```python
from build123d import *

# Parameters (mm, degrees)
SKETCH1_R                                    = 27
BOSS_EXTRUDE1_DEPTH                          = 4
CBORE_FOR_M3_HEX_SOCKET_THIN_HEAD_CA_2_COUNT = 2
CBORE_FOR_M3_HEX_SOCKET_THIN_HEAD_CA_2_PITCH = 31.112698372
CBORE_FOR_M3_HEX_SOCKET_THIN_HEAD_CA_3_COUNT = 2
CBORE_FOR_M3_HEX_SOCKET_THIN_HEAD_CA_3_PITCH = 44
CBORE_FOR_M3_HEX_SOCKET_THIN_HEAD_CA_4_COUNT = 2
CBORE_FOR_M3_HEX_SOCKET_THIN_HEAD_CA_4_PITCH = 31.112698372
BOSS_EXTRUDE2_START                          = -4
BOSS_EXTRUDE2_DEPTH                          = 4
SKETCH5_R                                    = 15
CUT_EXTRUDE1_DEPTH                           = 41.558599581


with BuildPart() as part:
    # Sketch1 → Boss-Extrude1 (new body)
    with BuildSketch(Plane.XY):
        Circle(SKETCH1_R)
    extrude(amount=BOSS_EXTRUDE1_DEPTH)

    # Sketch3 → CBORE for M3 Hex Socket Thin Head Cap Screw1 (revolve, cut)
    with BuildSketch(Plane(origin=(-22, 0, 4), x_dir=(0, -1, 0), z_dir=(1, 0, 0))):
        Polygon((0, 0), (0, 4), (1.7, 4), (1.7, 2.4), (3.25, 2.4), (3.25, 0.025), (3.275, 0), align=None)
    cbore_for_m3_hex_socket_thin_head_cap_sc = revolve(axis=Axis((-22, 0, 10.35), (0, 0, -1)), mode=Mode.SUBTRACT)

    # CBORE for M3 Hex Socket Thin Head Ca 2: CBORE for M3 Hex Socket Thin Head Cap Screw1 ×2
    with Locations(*[Vector(0.7071067811865277, 0.7071067811865674, 0) * (i * CBORE_FOR_M3_HEX_SOCKET_THIN_HEAD_CA_2_PITCH) for i in range(1, CBORE_FOR_M3_HEX_SOCKET_THIN_HEAD_CA_2_COUNT)]):
        add(cbore_for_m3_hex_socket_thin_head_cap_sc, mode=Mode.SUBTRACT)

    # CBORE for M3 Hex Socket Thin Head Ca 3: CBORE for M3 Hex Socket Thin Head Cap Screw1 ×2
    with Locations(*[(i * CBORE_FOR_M3_HEX_SOCKET_THIN_HEAD_CA_3_PITCH, 0, 0) for i in range(1, CBORE_FOR_M3_HEX_SOCKET_THIN_HEAD_CA_3_COUNT)]):
        add(cbore_for_m3_hex_socket_thin_head_cap_sc, mode=Mode.SUBTRACT)

    # CBORE for M3 Hex Socket Thin Head Ca 4: CBORE for M3 Hex Socket Thin Head Cap Screw1 ×2
    with Locations(*[Vector(0.7071067811865676, -0.7071067811865276, 0) * (i * CBORE_FOR_M3_HEX_SOCKET_THIN_HEAD_CA_4_PITCH) for i in range(1, CBORE_FOR_M3_HEX_SOCKET_THIN_HEAD_CA_4_COUNT)]):
        add(cbore_for_m3_hex_socket_thin_head_cap_sc, mode=Mode.SUBTRACT)

    # Sketch4 → Boss-Extrude2 (add)
    with BuildSketch(Plane.XY.offset(4).offset(BOSS_EXTRUDE2_START)):
        with BuildLine():
            Line((-27, 0), (-27, -30))
            Line((-27, -30), (27, -30))
            Line((27, -30), (27, 0))
            ThreePointArc((27, 0), (0, -27), (-27, 0))
        make_face()
    extrude(amount=BOSS_EXTRUDE2_DEPTH)

    # Sketch5 → Cut-Extrude1 (cut, through all)
    with BuildSketch(Plane(origin=(0, 0, 0), x_dir=(-1, 0, 0), z_dir=(0, 0, -1))):
        Circle(SKETCH5_R)
    extrude(amount=-CUT_EXTRUDE1_DEPTH, mode=Mode.SUBTRACT)


solid = part.part
```
Geometry check sheet. Reference: the model listing, model coordinates, mm. A direction names the side the tool comes from. Coordinates: 2 decimals unless noted, no trailing zeros. Order: outer loops, then holes, each group sorted by start corner. A loop starts at its lowest first (then second) coordinate and runs counter-clockwise, first axis right, second up.
Q1. Thickness scan on probe 1 along Y at (x, z) = (0, 3.3); probe 2 along Y at (x, z) = (0, 0.8); probe 3 along X at (y, z) = (0.5, 1.55). Record the ranges inside material, lowest first.
Reply:
probe 1: y = -30 to -25.25, -18.75 to -15, 15 to 18.75, 25.25 to 27
probe 2: y = -30 to -23.7, -20.3 to -15, 15 to 20.3, 23.7 to 27
probe 3: x = -27 to -23.62, -20.38 to -14.99, 14.99 to 20.38, 23.62 to 27
Q2. Depth check by flat-ended pin: pin 1 Ø3 at (x, y) = (23, 0.5) entering from +Z; pin 2 Ø7.5 at (x, y) = (-22, 0) entering from +Z. Enter the tip coordinate at first touch or a pass-through.
Reply:
pin 1: stops at z = 1.6
pin 2: stops at z = 4
Q3. Tool access check on faces 4 (the face through (-6, -14, 4)), 5 (the face through (-0.98, 18.9, 2.8)). Record the directions out of +Z, -Z, +X, -X, +Y, -Y that give a thin tool (end or side, any length) a straight path to the whole face; none if there is none.
Reply:
face 4: +Z, +X, -X, +Y, -Y
face 5: +Z
Q4. Sectioned sample at C-C on x = 10.5. Record the cut outline in (y, z), and give its area (3 significant figures).
Reply:
outline: (-30, 0) - (-10.71, 0) - (-10.71, 4) - (-30, 4) - close; (10.71, 0) - (24.87, 0) - (24.87, 4) - (10.71, 4) - close
area: 134 mm2
Q5. Sectioned sample at A-A on x = 0. Record the cut outline in (y, z) (3 decimals).
Reply:
outline: (-30, 0) - (-23.7, 0) - (-23.7, 1.6) - (-25.25, 1.6) - (-25.25, 3.975) - (-25.275, 4) - (-30, 4) - close; (-20.3, 0) - (-15, 0) - (-15, 4) - (-18.725, 4) - (-18.75, 3.975) - (-18.75, 1.6) - (-20.3, 1.6) - close; (15, 0) - (20.3, 0) - (20.3, 1.6) - (18.75, 1.6) - (18.75, 3.975) - (18.725, 4) - (15, 4) - close; (23.7, 0) - (27, 0) - (27, 4) - (25.275, 4) - (25.25, 3.975) - (25.25, 1.6) - (23.7, 1.6) - close
Q6. Sectioned sample at D-D on y = 7. Record the cut outline in (x, z), and give its area (3 significant figures).
Reply:
outline: (-26.08, 0) - (-13.27, 0) - (-13.27, 4) - (-26.08, 4) - close; (13.27, 0) - (26.08, 0) - (26.08, 4) - (13.27, 4) - close
area: 102 mm2
Q7. Draft check along X on faces 1 (the face through (-0.143, -18.753, 2.804)), 2 (the face through (-6, -14, 0)), 3 (the face through (27, -15, 2)). Enter one of: released by +X, released by -X, zero draft, split by the parting line, or undercut.
Reply:
face 1: undercut
face 2: zero draft
face 3: released by +X
Q8. Sectioned sample at B-B on y = -22. Record the cut outline in (x, z) (3 decimals), and give its area (3 significant figures).
Reply:
outline: (-27, 0) - (-1.7, 0) - (-1.7, 1.6) - (-3.25, 1.6) - (-3.25, 3.975) - (-3.275, 4) - (-27, 4) - close; (1.7, 0) - (27, 0) - (27, 4) - (3.275, 4) - (3.25, 3.975) - (3.25, 1.6) - (1.7, 1.6) - close
area: 195 mm2
